Input: dimensioned drawing with shaded views. Units: mm. Origin: part minimum x, y, z. A direction names the side the tool comes from. Give positions to 0.01 mm unless a question says otherwise; leave off trailing zeros. Write each loop counter-clockwise with the first axis right and the second up, starting at its lowest first coordinate (ties: lowest second). Pieces come first, ordered by that corner, then holes.
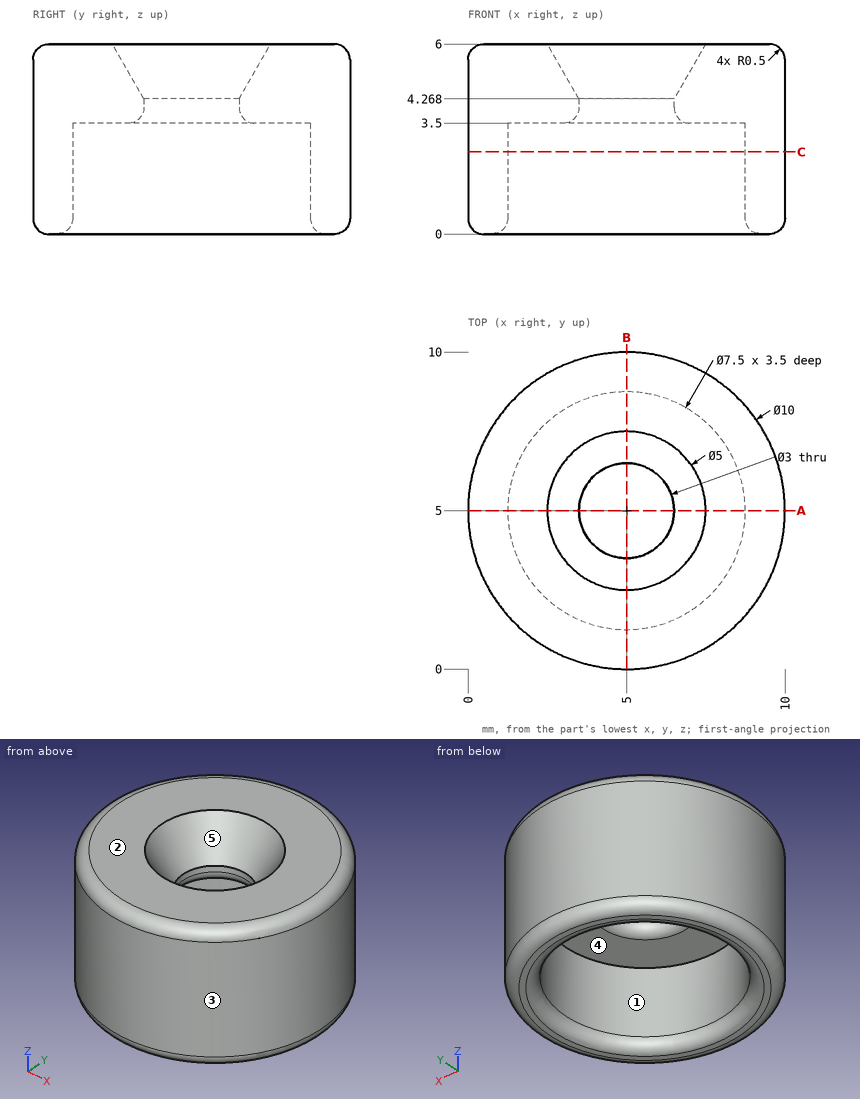
Item 1: Pull-direction query (X, two-part tool) for the marked faces 1, 2 and 3; classes: +X half, -X half, draft (parallel to the pull), parting line (faces both ways), or undercut.
Found:
face 1: undercut
face 2: draft
face 3: parting line
Item 2: Pin query (flat end, axial travel): pin 1 Ø1.5 at (x, z) = (8, 1.5) entering from +Y (3 decimals); pin 2 Ø1 at (y, z) = (8.5, 1) entering from +X; pin 3 Ø1 at (y, z) = (6, 3) entering from -X (3 decimals); pin 4 Ø3 at (y, z) = (6.5, 2) entering from +X. Return the tip coordinate at first contact, or that it passes through.
Found:
pin 1: stops at y = 9.465
pin 2: stops at x = 9
pin 3: stops at x = 0.025
pin 4: stops at x = 10
Item 3: Section A-A, the plane y = 5. Return the cut outline in (x, z).
Found:
outline: (0, 0.5) arc R0.5 ccw to (0.5, 0) - (0.75, 0) arc R0.5 ccw to (1.25, 0.5) - (1.25, 3.5) - (3, 3.5) arc R0.5 ccw to (3.5, 4) - (3.5, 4.27) - (2.5, 6) - (0.5, 6) arc R0.5 ccw to (0, 5.5) - close; (6.5, 4) arc R0.5 ccw to (7, 3.5) - (8.75, 3.5) - (8.75, 0.5) arc R0.5 ccw to (9.25, 0) - (9.5, 0) arc R0.5 ccw to (10, 0.5) - (10, 5.5) arc R0.5 ccw to (9.5, 6) - (7.5, 6) - (6.5, 4.27) - close
Item 4: Line query: L1, parallel to Y at x = 5, z = 4.2; L2, parallel to Y at x = 5, z = 2.85; L3, parallel to Z at x = 1.75, y = 6.5. Output: solid intervals per line, ascending.
Found:
L1: y = 0 to 3.5, 6.5 to 10
L2: y = 0 to 1.25, 8.75 to 10
L3: z = 3.5 to 6
Item 5: Section C-C, the plane z = 2.6. Return the cut outline in (x, y), plus the area to 3 significant figures.
Found:
outline: circle Ø10 at (5, 5); hole circle Ø7.5 at (5, 5)
area: 34.4 mm2
Item 6: Reachability of the marked faces 4 and 5 from +Z, -Z, +X, -X, +Y, -Y: full face, straight path, thin tool, end or side. Return the list, or none.
Found:
face 4: -Z
face 5: +Z
